from build123d import *

# Parameters (mm, degrees)
BOSS_EXTRUDE1_DEPTH   = 10
FILLET1_R             = 3
F_3_0MM_DOWEL_HOLE1_D = 3


with BuildPart() as part:
    # Sketch1 → Boss-Extrude1 (new body)
    with BuildSketch(Plane.XY):
        Polygon((0, -20.5), (0, 20.5), (-21, 20.5), (-21, 32.5), (5, 32.5), (5, -32.5), (-21, -32.5), (-21, -20.5), align=None)
    extrude(amount=BOSS_EXTRUDE1_DEPTH)

    # Fillet1
    fillet1_edges = [part.edges().sort_by_distance(p)[0] for p in [
        (0, -20.5, 5),
        (0, 20.5, 5),
        (-21, 20.5, 5),
        (-21, 32.5, 5),
        (5, 32.5, 5),
        (5, -32.5, 5),
        (-21, -32.5, 5),
        (-21, -20.5, 5),
    ]]
    fillet(fillet1_edges, radius=FILLET1_R)

    # Ø3.0mm Dowel Hole1 (through all)
    with Locations(Plane.XY.offset(10)):
        with Locations((-5.3, 24.695), (-15.2, 24.695)):
            f_3_0mm_dowel_hole1 = Hole(F_3_0MM_DOWEL_HOLE1_D / 2)

    # Mirror1: Ø3.0mm Dowel Hole1 across plane
    add(f_3_0mm_dowel_hole1.mirror(Plane.ZX), mode=Mode.SUBTRACT)


solid = part.part
Check sheet for the modelled part. Datum: model origin and axes. Units: mm. A direction names the side the tool comes from. Give positions to 0.01 mm unless a question says otherwise; leave off trailing zeros. Loops run counter-clockwise (first coordinate to the right, second up) from the corner with the lowest first, then second, coordinate; pieces in that order, holes last. Notation, with made-up numbers: M -17.5,-4 L 39.5,-4 A16 ccw 39.5,23 Z; hole C -35.5,21 d11. An arc over 180 degrees is marked long. Answer as a JSON object with one key per item and string values. Group by question number.
Q1. Cross-section at C-C on z = 4. Record the cut outline in (x, y) (3 decimals).
Q2. Cross-section at B-B on x = -15.2. Record the cut outline in (y, z) (3 decimals).
Q3. Cross-section at D-D on y = -8. Record the cut outline in (x, z), then the cut area to 3 significant figures.
Q4. Material ranges on line 1 along Y through (x, z) = (-15.2, 3) (3 decimals); line 2 along Y through (x, z) = (-6, 6); line 3 along Y through (x, z) = (-18.25, 0.5), recorded low to high. Write a range as [from, to].
Q5. Cross-section at A-A on x = -12.5. Record the cut outline in (y, z), then the cut area to 3 significant figures.
Q6. Release check for a two-part mould opening along Y. For faces 3 (the cylindrical face through (-20.1, 21.36, 5.07)), 4 (the flat face through (5, 0, 5)), 5 (the cylindrical face through (-20.14, 31.6, 5.07)) record: released by +Y, released by -Y, zero draft, split by the parting line, or undercut.
Q7. Go/stop test with flat-tipped pins: P1, Ø2.5, axis at x = -5.3, y = -24.695, coming from the -Z side; P2, Ø1, axis at y = -5, z = 3.5, coming from the -X side. Record where each tip stops, or that it passes through.
Q8. Access from +Z, -Z, +X, -X, +Y, -Y to the whole of each face (thin tool, end or side, straight path). Record for faces 1 (the flat face through (-21, -27, 5)), 2 (the flat face through (-10, 20.5, 5)).
Evaluation:
{
 "1": {"outline": "M -21,-29.5 A3 ccw -18,-32.5 L 2,-32.5 A3 ccw 5,-29.5 L 5,29.5 A3 ccw 2,32.5 L -18,32.5 A3 ccw -21,29.5 L -21,23.5 A3 ccw -18,20.5 L -3,20.5 A3 cw 0,17.5 L 0,-17.5 A3 cw -3,-20.5 L -18,-20.5 A3 ccw -21,-23.5 Z; hole C -15.2,-24.695 d3; hole C -15.2,24.695 d3; hole C -5.3,-24.695 d3; hole C -5.3,24.695 d3"},
 "2": {"outline": "M -32.5,0 L -26.195,0 L -26.195,10 L -32.5,10 Z; M -23.195,0 L -20.5,0 L -20.5,10 L -23.195,10 Z; M 20.5,0 L 23.195,0 L 23.195,10 L 20.5,10 Z; M 26.195,0 L 32.5,0 L 32.5,10 L 26.195,10 Z"},
 "3": {"outline": "M 0,0 L 5,0 L 5,10 L 0,10 Z", "area": "50.0 mm2"},
 "4": {"line 1": "y = [-32.5, -26.195], [-23.195, -20.5], [20.5, 23.195], [26.195, 32.5]", "line 2": "y = [-32.5, -26.02], [-23.37, -20.5], [20.5, 23.37], [26.02, 32.5]", "line 3": "y = [-32.49, -20.51], [20.51, 32.49]"},
 "5": {"outline": "M -32.5,0 L -20.5,0 L -20.5,10 L -32.5,10 Z; M 20.5,0 L 32.5,0 L 32.5,10 L 20.5,10 Z", "area": "240 mm2"},
 "6": {"face 3": "undercut", "face 4": "zero draft", "face 5": "released by +Y"},
 "7": {"P1": "passes through", "P2": "stops at x = 0"},
 "8": {"face 1": "+Z, -Z, -X, +Y, -Y", "face 2": "+Z, -Z, -X"}
}
